The model under review builds one solid part; all positions refer to its coordinate system, in mm. Face numbers are marked on the shaded views. Coordinates: 2 decimals unless noted, no trailing zeros. Loops run counter-clockwise (first coordinate to the right, second up) from the corner with the lowest first, then second, coordinate; pieces in that order, holes last. Notation, with made-up numbers: (29.5, -38.5) - (52.5, -38.5) arc R22 cw to (52.5, -32.5) - close; hole circle Ø11 at (86, 15.25). An arc over 180 degrees is marked (long way). One line per item, written item: value. Start each with the question number.
1. Mouldability with a two-part tool opening along X and no side actions: class the marked faces 1 and 2 as +X half, -X half, draft (parallel to the pull), parting line (faces both ways), or undercut.
2. Insertion check: P1, Ø1.9, axis at y = 2.5, z = 15, coming from the +X side; P2, Ø1.1, axis at y = 1, z = 14, coming from the -X side; P3, Ø4, axis at x = -8.5, z = -16.5, coming from the +Y side; P4, Ø1, axis at y = 2, z = 5, coming from the -X side. Each pin has a flat end and moves straight along its axis. Give the tip position at first contact, or say it passes through.
3. We need section C-C, the plane z = -12.5. Give the boundary of the cut face in (x, y), then the cut area to 3 significant figures.
4. To check wall thickness, follow line 1 (X direction, y = 3.25, z = -24); line 2 (X direction, y = 2.5, z = 11.5); line 3 (X direction, y = 2.65, z = -0.5). State the ranges of each line that lie inside material, in increasing order.
5. We need section B-B, the plane x = 0. Give the boundary of the cut face in (y, z), then the cut area to 3 significant figures.
6. We need section D-D, the plane x = 11. Give the boundary of the cut face in (y, z), then the cut area to 3 significant figures.
7. We need section A-A, the plane y = 2.9. Give the boundary of the cut face in (x, z) (3 decimals).
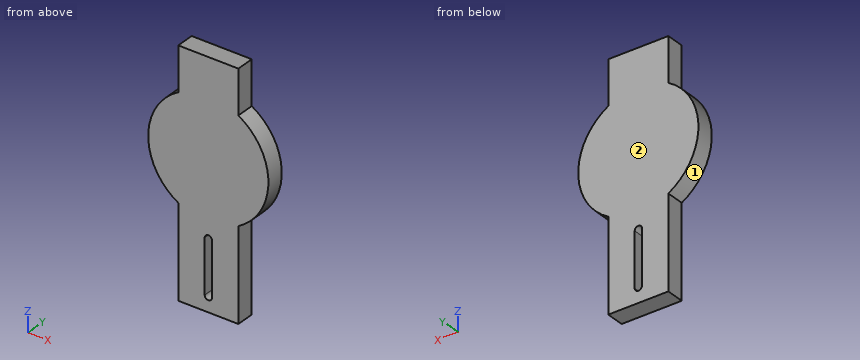
from build123d import *

# Parameters (mm, degrees)
BOSS_EXTRUDE1_DEPTH = 3.81


with BuildPart() as part:
    # Sketch2 → Boss-Extrude1 (new body)
    with BuildSketch(Plane(origin=(0, 0, 0), x_dir=(1, 0, 0), z_dir=(0, 1, 0))):
        with BuildLine():
            Line((6.35, 10.998522628), (6.35, 30.48))
            Line((6.35, 30.48), (-6.35, 30.48))
            Line((-6.35, 30.48), (-6.35, 10.998522628))
            ThreePointArc((-6.35, 10.998522628), (-12.7, 0), (-6.35, -10.998522628))
            Line((-6.35, -10.998522628), (-6.35, -20.32))
            Line((-6.35, -20.32), (6.35, -20.32))
            Line((6.35, -20.32), (6.35, -10.998522628))
            ThreePointArc((6.35, -10.998522628), (12.7, 0), (6.35, 10.998522628))
        make_face()
        with BuildLine():
            Line((-0.762, 15.875), (-0.762, 27.305))
            ThreePointArc((-0.762, 27.305), (0, 28.067), (0.762, 27.305))
            Line((0.762, 27.305), (0.762, 15.875))
            ThreePointArc((0.762, 15.875), (0, 15.113), (-0.762, 15.875))
        make_face(mode=Mode.SUBTRACT)
    extrude(amount=BOSS_EXTRUDE1_DEPTH)


solid = part.part
Findings below:
1. face 1: -X half
1. face 2: draft
2. P1: x = 6.35
2. P2: x = -6.35
2. P3: through
2. P4: x = -11.88
3. outline: (-6.35, 0) - (6.35, 0) - (6.35, 3.81) - (-6.35, 3.81) - close
3. area: 48.4 mm2
4. line 1: -6.35 to -0.76, 0.76 to 6.35
4. line 2: -6.35 to 6.35
4. line 3: -12.69 to 12.69
5. outline: (0, -30.48) - (3.81, -30.48) - (3.81, -28.07) - (0, -28.07) - close; (0, -15.11) - (3.81, -15.11) - (3.81, 20.32) - (0, 20.32) - close
5. area: 144 mm2
6. outline: (0, -6.35) - (3.81, -6.35) - (3.81, 6.35) - (0, 6.35) - close
6. area: 48.4 mm2
7. outline: (-6.35, -30.48) - (6.35, -30.48) - (6.35, -10.999) arc R12.7 ccw to (6.35, 10.999) - (6.35, 20.32) - (-6.35, 20.32) - (-6.35, 10.999) arc R12.7 ccw to (-6.35, -10.999) - close; hole (-0.762, -27.305) arc R0.762 ccw to (0.762, -27.305) - (0.762, -15.875) arc R0.762 ccw to (-0.762, -15.875) - close
